from build123d import *

# Parameters (mm, degrees)
SKETCH1_W             = 38.1
SKETCH1_H             = 38.1
BOSS_EXTRUDE1_DEPTH   = 457.2
BOSS_EXTRUDE1_2_DEPTH = 457.2
SKETCH2_W             = 25.4
SKETCH2_H             = 25.4
BOSS_EXTRUDE2_DEPTH   = 521.97
BOSS_EXTRUDE3_START   = 431.8
SKETCH3_R             = 6.35
BOSS_EXTRUDE3_DEPTH   = 25.4


with BuildPart() as part:
    # Sketch1 → Boss-Extrude1 (new body)
    with BuildSketch(Plane(origin=(0, 0, 0), x_dir=(1, 0, 0), z_dir=(0, 1, 0))):
        with Locations((-260.35, 0)):
            Rectangle(SKETCH1_W, SKETCH1_H)
    extrude(amount=BOSS_EXTRUDE1_DEPTH)



with BuildPart() as body_2:
    # Sketch1 → Boss-Extrude1 2 (new body)
    with BuildSketch(Plane(origin=(0, 0, 0), x_dir=(1, 0, 0), z_dir=(0, 1, 0))):
        with Locations((260.35, 0)):
            Rectangle(SKETCH1_W, SKETCH1_H)
    extrude(amount=BOSS_EXTRUDE1_2_DEPTH)


with BuildPart() as part_1:
    add(part.part)

    add(body_2.part)  # Boss-Extrude2 merges body 2
    # Sketch2 → Boss-Extrude2 (add)
    with BuildSketch(Plane(origin=(279.4, 0, 0), x_dir=(0, 0, -1), z_dir=(1, 0, 0))):
        with Locations((0, 419.1)):
            Rectangle(SKETCH2_W, SKETCH2_H)
    extrude(amount=-BOSS_EXTRUDE2_DEPTH)

    # Sketch3 → Boss-Extrude3 (add)
    with BuildSketch(Plane(origin=(0, 0, 0), x_dir=(1, 0, 0), z_dir=(0, 1, 0)).offset(BOSS_EXTRUDE3_START)):
        with Locations(Location((0, 0, 0), (0, 0, 270))):
            Circle(SKETCH3_R)
    extrude(amount=BOSS_EXTRUDE3_DEPTH)


solid = part_1.part
Read the model definition and answer for the solid it produces. Units are mm, in the model's axes. A direction names the side the tool comes from. Round coordinates to 2 decimals unless told otherwise and drop trailing zeros. Write each loop counter-clockwise with the first axis right and the second up, starting at its lowest first coordinate (ties: lowest second). Pieces come first, ordered by that corner, then holes.
1. Determine the mould class of faces 4 (the face through (260, 225, -19.05)), 5 (the face through (241.3, 225, 0)), 6 (the face through (-279.4, 225, 0)) for opening direction X: pulls with the +X half, pulls with the -X half, needs draft (parallel to the pull), parting line crosses it, or undercut.
2. Which of the six approach directions +Z, -Z, +X, -X, +Y, -Y give full straight-line access (tool end or side, diameter ignored) to faces 1 (the face through (3, 419, 12.7)), 2 (the face through (3, 419, -12.7)), 3 (the face through (3, 406.4, 0))?
3. Straight lines are drawn through the part: L1, parallel to X at y = 73, z = -5.5; L2, parallel to Y at x = -206, z = -11.5; L3, parallel to Z at x = -80, y = 424.5. For each, find the intervals that lie inside material, in ascending order.
4. The part is cut by section A-A, the plane y = 280.5. Determine the outline of the cut face in (x, z), then the cut area to 3 significant figures.
5. Given pin 1 Ø7.5 at (x, y) = (34, 422.5) entering from -Z; pin 2 Ø7.5 at (x, y) = (2, 421) entering from +Z; pin 3 Ø2 at (x, z) = (-159, -5) entering from +Y, each flat-ended and moving along its own axis, determine where each tip first touches the part or whether it passes through.
6. The part is cut by section C-C, the plane z = 0. Determine the outline of the cut face in (x, y), then the cut area to 3 significant figures.
7. The part is cut by section B-B, the plane x = 0. Determine the outline of the cut face in (y, z).
Values:
1. face 4: needs draft
1. face 5: undercut
1. face 6: pulls with the -X half
2. face 1: +Z, +Y, -Y
2. face 2: -Z, +Y, -Y
2. face 3: +Z, -Z, -Y
3. L1: x = -279.4 to -241.3, 241.3 to 279.4
3. L2: y = 406.4 to 431.8
3. L3: z = -12.7 to 12.7
4. outline: (-279.4, -19.05) - (-241.3, -19.05) - (-241.3, 19.05) - (-279.4, 19.05) - close; (241.3, -19.05) - (279.4, -19.05) - (279.4, 19.05) - (241.3, 19.05) - close
4. area: 2,900 mm2
5. pin 1: stops at z = -12.7
5. pin 2: stops at z = 12.7
5. pin 3: stops at y = 431.8
6. outline: (-279.4, 0) - (-241.3, 0) - (-241.3, 406.4) - (241.3, 406.4) - (241.3, 0) - (279.4, 0) - (279.4, 457.2) - (241.3, 457.2) - (241.3, 431.8) - (6.35, 431.8) - (6.35, 457.2) - (-6.35, 457.2) - (-6.35, 431.8) - (-241.3, 431.8) - (-241.3, 457.2) - (-279.4, 457.2) - close
6. area: 47,400 mm2
7. outline: (406.4, -12.7) - (431.8, -12.7) - (431.8, -6.35) - (457.2, -6.35) - (457.2, 6.35) - (431.8, 6.35) - (431.8, 12.7) - (406.4, 12.7) - close
